```python
from build123d import *

# Parameters (mm, degrees)
F0_W     = 7
F0_H     = 11
F1_DEPTH = 7
F2_R     = 1.5
F3_DEPTH = 7.001
F4_R     = 1.5
F5_DEPTH = 25


with BuildPart() as f1:
    # F0 (on Top) → F1 (new body)
    with BuildSketch(Plane.XY):
        Rectangle(F0_W, F0_H)
    extrude(amount=F1_DEPTH)

    # F2 (on face) → F3 (cut, through all)
    with BuildSketch(Plane.XY.offset(7)):
        with Locations((0, 2)):
            Circle(F2_R)
    extrude(amount=-F3_DEPTH, mode=Mode.SUBTRACT)

    # F4 (on face) → F5 (cut)
    with BuildSketch(Plane(origin=(-3.5, 0, 0), x_dir=(0, -1, 0), z_dir=(-1, 0, 0))):
        with Locations((2, 3.5)):
            Circle(F4_R)
    extrude(amount=-F5_DEPTH, mode=Mode.SUBTRACT)


solid = f1.part
```
Read the model definition and answer for the solid it produces. Units are mm, in the model's axes. Round coordinates to 2 decimals unless told otherwise and drop trailing zeros. Write each loop counter-clockwise with the first axis right and the second up, starting at its lowest first coordinate (ties: lowest second). Pieces come first, ordered by that corner, then holes. Notation, with made-up numbers: (62, -4.75) - (110, -4.75) arc R25 ccw to (110, 12.25) - close; hole circle Ø6 at (38, 49.25). An arc over 180 degrees is marked (long way). One line per item, written item: value.
Q1. Find section B-B (x = 0). Determine the outline of the cut face in (y, z).
The answers:
outline: (-5.5, 0) - (0.5, 0) - (0.5, 7) - (-5.5, 7) - close; (3.5, 0) - (5.5, 0) - (5.5, 7) - (3.5, 7) - close; hole circle Ø3 at (-2, 3.5)
Q2. Find section D-D (x = 2.5). Determine the outline of the cut face in (y, z), and give its area (3 significant figures).
The answers:
outline: (-5.5, 0) - (5.5, 0) - (5.5, 7) - (-5.5, 7) - close; hole circle Ø3 at (-2, 3.5)
area: 69.9 mm2
Q3. Straight lines are drawn through the part: line 1 (Z direction, x = -2.75, y = -2); line 2 (Y direction, x = -1, z = 6.25); line 3 (Y direction, x = 2.75, z = 3). For each, find the intervals that lie inside material, in ascending order. Write a range as from..to.
The answers:
line 1: z = 0..2, 5..7
line 2: y = -5.5..0.88, 3.12..5.5
line 3: y = -5.5..-3.41, -0.59..5.5
Q4. Find section A-A (z = 3.5). Determine the outline of the cut face in (x, y), and give its area (3 significant figures).
The answers:
outline: (-3.5, -5.5) - (3.5, -5.5) - (3.5, -3.5) - (-3.5, -3.5) - close; (-3.5, -0.5) - (3.5, -0.5) - (3.5, 5.5) - (-3.5, 5.5) - close; hole circle Ø3 at (0, 2)
area: 48.9 mm2
Q5. For a pull along Z with two mould halves and no side action, classify faces 1 (the cylindrical face through (-0.05, -0.5, 3.57)), 2 (the flat face through (-3.5, 0, 3)), 3 (the flat face through (0, 0, 7)) as pulls with the +Z half, pulls with the -Z half, needs draft (parallel to the pull), parting line crosses it, or undercut.
The answers:
face 1: undercut
face 2: needs draft
face 3: pulls with the +Z half
Q6. Find section C-C (y = 2). Determine the outline of the cut face in (x, z).
The answers:
outline: (-3.5, 0) - (-1.5, 0) - (-1.5, 7) - (-3.5, 7) - close; (1.5, 0) - (3.5, 0) - (3.5, 7) - (1.5, 7) - close
